```python
from build123d import *

# Parameters (mm, degrees)
CROQUIS1_W              = 50
CROQUIS1_H              = 76
SALIENTE_EXTRUIR1_DEPTH = 28
CROQUIS2_R              = 2
CORTAR_EXTRUIR1_DEPTH   = 28
CROQUIS3_W              = 51.795240056
CROQUIS3_H              = 77.113165798
SALIENTE_EXTRUIR2_DEPTH = 1
CROQUIS4_W              = 3.63093588
CROQUIS4_H              = 19.245174354
CORTAR_EXTRUIR2_DEPTH   = 10
SALIENTE_EXTRUIR3_DEPTH = 3.2
CROQUIS6_R              = 0.9
CORTAR_EXTRUIR3_DEPTH   = 10
CORTAR_EXTRUIR4_DEPTH   = 10


with BuildPart() as part:
    # Croquis1 → Saliente-Extruir1 (new body)
    with BuildSketch(Plane.XY):
        with BuildLine():
            Line((-24, 41), (-22.544096538, 41))
            Line((-22.544096538, 41), (-22.544096538, 44.762632311))
            Line((-22.544096538, 44.762632311), (-15.074666962, 44.762632311))
            Line((-15.074666962, 44.762632311), (-15.074666962, 41))
            Line((-15.074666962, 41), (15.074666962, 41))
            Line((15.074666962, 41), (15.074666962, 44.762632311))
            Line((15.074666962, 44.762632311), (22.544096538, 44.762632311))
            Line((22.544096538, 44.762632311), (22.544096538, 41))
            Line((22.544096538, 41), (24, 41))
            ThreePointArc((24, 41), (26.828427125, 39.828427125), (28, 37))
            Line((28, 37), (28, -37))
            ThreePointArc((28, -37), (26.828427125, -39.828427125), (24, -41))
            Line((24, -41), (22.544096538, -41))
            Line((22.544096538, -41), (22.544096538, -44.762632311))
            Line((22.544096538, -44.762632311), (15.074666962, -44.762632311))
            Line((15.074666962, -44.762632311), (15.074666962, -41))
            Line((15.074666962, -41), (-15.074666962, -41))
            Line((-15.074666962, -41), (-15.074666962, -44.762632311))
            Line((-15.074666962, -44.762632311), (-22.544096538, -44.762632311))
            Line((-22.544096538, -44.762632311), (-22.544096538, -41))
            Line((-22.544096538, -41), (-24, -41))
            ThreePointArc((-24, -41), (-26.828427125, -39.828427125), (-28, -37))
            Line((-28, -37), (-28, 37))
            ThreePointArc((-28, 37), (-26.828427125, 39.828427125), (-24, 41))
        make_face()
        Rectangle(CROQUIS1_W, CROQUIS1_H, mode=Mode.SUBTRACT)
    extrude(amount=SALIENTE_EXTRUIR1_DEPTH)

    # Croquis2 → Cortar-Extruir1 (cut)
    with BuildSketch(Plane.XY.offset(28)):
        with Locations((-19, 41.25)):
            Circle(CROQUIS2_R)
        with Locations((19, 41.25)):
            Circle(CROQUIS2_R)
        with Locations((-19, -41.25)):
            Circle(CROQUIS2_R)
        with Locations((19, -41.25)):
            Circle(CROQUIS2_R)
    extrude(amount=-CORTAR_EXTRUIR1_DEPTH, mode=Mode.SUBTRACT)

    # Croquis3 → Saliente-Extruir2 (add)
    with BuildSketch(Plane(origin=(0, 0, 0), x_dir=(-1, 0, 0), z_dir=(0, 0, -1))):
        Rectangle(CROQUIS3_W, CROQUIS3_H)
    extrude(amount=-SALIENTE_EXTRUIR2_DEPTH)

    # Croquis4 → Cortar-Extruir2 (cut)
    with BuildSketch(Plane(origin=(0, 0, 0), x_dir=(-1, 0, 0), z_dir=(0, 0, -1))):
        with Locations((23.544656322, 14.5)):
            Rectangle(CROQUIS4_W, CROQUIS4_H)
    extrude(amount=-CORTAR_EXTRUIR2_DEPTH, mode=Mode.SUBTRACT)

    # Croquis5 → Saliente-Extruir3 (add)
    with BuildSketch(Plane.XY.offset(1)):
        with BuildLine():
            Line((8.6, -32.204355183), (8.6, -11.804355183))
            ThreePointArc((8.6, -11.804355183), (6.6, -9.804355183), (4.6, -11.804355183))
            Line((4.6, -11.804355183), (4.6, -32.204355183))
            ThreePointArc((4.6, -32.204355183), (6.6, -34.204355183), (8.6, -32.204355183))
        make_face()
    extrude(amount=SALIENTE_EXTRUIR3_DEPTH)

    # Croquis6 → Cortar-Extruir3 (cut)
    with BuildSketch(Plane.XY.offset(4.2)):
        with Locations((6.6, -32.204355183)):
            Circle(CROQUIS6_R)
        with Locations((6.6, -11.804355183)):
            Circle(CROQUIS6_R)
    extrude(amount=-CORTAR_EXTRUIR3_DEPTH, mode=Mode.SUBTRACT)

    # Croquis7 → Cortar-Extruir4 (cut)
    with BuildSketch(Plane.ZY.offset(28)):
        with BuildLine():
            Line((3.589785913, -27.724097248), (1.561156319, -27.724097248))
            ThreePointArc((1.561156319, -27.724097248), (0.146942756, -27.13831081), (-0.438843681, -25.724097248))
            Line((-0.438843681, -25.724097248), (-0.438843681, -18.821747943))
            ThreePointArc((-0.438843681, -18.821747943), (0.146942756, -17.407534381), (1.561156319, -16.821747943))
            Line((1.561156319, -16.821747943), (3.589785913, -16.821747943))
            ThreePointArc((3.589785913, -16.821747943), (5.003999475, -17.407534381), (5.589785913, -18.821747943))
            Line((5.589785913, -18.821747943), (5.589785913, -25.724097248))
            ThreePointArc((5.589785913, -25.724097248), (5.003999475, -27.13831081), (3.589785913, -27.724097248))
        make_face()
    extrude(amount=-CORTAR_EXTRUIR4_DEPTH, mode=Mode.SUBTRACT)


solid = part.part
```
Model file for the job. Use its own axes, mm. A direction names the side the tool comes from. Give positions to 0.01 mm unless a question says otherwise; leave off trailing zeros. Order: outer loops, then holes, each group sorted by start corner. A loop starts at its lowest first (then second) coordinate and runs counter-clockwise, first axis right, second up.
1) Saw through at D-D, the plane x = -9.5. Write the cut outline in (y, z).
2) Saw through at C-C, the plane x = -19. Write the cut outline in (y, z).
3) Saw through at B-B, the plane z = 26. Count the separate pieces of the cut face and the enclosed holes in it, then the cut area to 3 significant figures.
4) Saw through at A-A, the plane x = 19. Write the cut outline in (y, z).
5) 3-axis set-ups, long thin cutter, end or side, ignore diameter. For faces 4 (the flat face through (-22.544, 43, 14)), 5 (the flat face through (7, -22, 4.2)), 6 (the flat face through (-15.075, -43, 14)): which of +Z, -Z, +X, -X, +Y, -Y reach the whole face in a straight line?
6) Mould opens along Z. For faces 1 (the cylindrical face through (-26.521, -17.392, 4.988)), 2 (the cylindrical face through (-26.859, 39.797, 13.804)), 3 (the flat face through (0, 1, 0)) say: +Z half, -Z half, draft (parallel to the pull), parting line (faces both ways), or undercut.
7) Pin check, flat tips, straight feed: pin 1 (2 mm diameter, centred on x = 5.5, y = -23.5, fed in from +Z); pin 2 (1.5 mm diameter, centred on x = -3.5, z = 21.5, fed in from +Y); pin 3 (3 mm diameter, centred on y = 43.5, z = 19.5, fed in from +X). Stop position of each tip, or through.
8) Wall check: probe 1 along Y at (x, z) = (19, 22.5); probe 2 along Y at (x, z) = (6.6, 1.55); probe 3 along X at (y, z) = (41.5, 2.75). Give the ranges that are in metal, low to high.
Computed:
1. outline: (-41, 0) - (41, 0) - (41, 28) - (38, 28) - (38, 1) - (-38, 1) - (-38, 28) - (-41, 28) - close
2. outline: (-44.76, 0) - (-43.25, 0) - (-43.25, 28) - (-44.76, 28) - close; (-39.25, 0) - (-26.97, 0) arc R2 cw to (-27.64, 1) - (-38, 1) - (-38, 28) - (-39.25, 28) - close; (-17.57, 0) - (39.25, 0) - (39.25, 28) - (38, 28) - (38, 1) - (-16.9, 1) arc R2 cw to start; (43.25, 0) - (44.76, 0) - (44.76, 28) - (43.25, 28) - close
3. separate pieces: 1
3. enclosed holes: 5
3. area: 840 mm2
4. outline: (-44.76, 0) - (-43.25, 0) - (-43.25, 28) - (-44.76, 28) - close; (-39.25, 0) - (39.25, 0) - (39.25, 28) - (38, 28) - (38, 1) - (-38, 1) - (-38, 28) - (-39.25, 28) - close; (43.25, 0) - (44.76, 0) - (44.76, 28) - (43.25, 28) - close
5. face 4: +Z, -Z, -X, +Y
5. face 5: +Z
5. face 6: +Z, -Z, -Y
6. face 1: undercut
6. face 2: draft
6. face 3: -Z half
7. pin 1: stops at z = 4.2
7. pin 2: stops at y = 41
7. pin 3: stops at x = 22.54
8. probe 1: y = -44.76 to -43.25, -39.25 to -38, 38 to 39.25, 43.25 to 44.76
8. probe 2: y = -41 to -38, -34.2 to -33.1, -31.3 to -12.7, -10.9 to -9.8, 38 to 41
8. probe 3: x = -22.54 to -20.98, -17.02 to -15.07, 15.07 to 17.02, 20.98 to 22.54
